Geometry check sheet. Reference: the model listing, model coordinates, mm. Round coordinates to 2 decimals unless told otherwise and drop trailing zeros. Loops run counter-clockwise (first coordinate to the right, second up) from the corner with the lowest first, then second, coordinate; pieces in that order, holes last. Notation, with made-up numbers: (62, 84.5) -> (74, 84.5) arc R16 ccw to (74, 107.5) -> close; hole circle Ø7 at (43.5, -29.5). An arc over 180 degrees is marked (long way). Use a Markdown table: item, result. Add a question column.
Q1. Sectioned sample at B-B, the plane y = 44.5. Enter the section's corners in (x, z).
Q2. Sectioned sample at A-A, the plane x = 13.75. Enter the section's corners in (y, z).
Q3. Material ranges on L1, parallel to Z at x = 18.5, y = 37; L2, parallel to Z at x = 12.5, y = 48; L3, parallel to X at y = 27, z = 25.5, recorded low to high.
Q4. Sectioned sample at C-C, the plane z = 31. Enter the section's corners in (x, y).
Q5. Gauge pin test, flat ends, axial feed: P1, Ø5.5, axis at y = 37, z = 24, coming from the -X side; P2, Ø1.5, axis at x = 19.5, y = 60, coming from the -Z side. Record the tip position at first contact, or that the pin passes through.
```python
from build123d import *

# Parameters (mm, degrees)
F1_DEPTH = 76.2
F2_R     = 5.08


with BuildPart() as f1:
    # F0 (on Front) → F1 (new body)
    with BuildSketch(Plane.XZ):
        Polygon((11.069345, -64.862475), (30.119345, -65.090583), (30.119345, 61.909417), (11.069345, 61.909417), (11.069345, 36.509417), (20.594345, 36.509417), (20.594345, 17.459417), (11.069345, 17.459417), align=None)
    extrude(amount=-F1_DEPTH)

    # F2
    f2_edges = [f1.edges().sort_by_distance(p)[0] for p in [
        (20.594345, 76.2, 61.909417),
        (30.119345, 38.1, 61.909417),
        (20.594345, 0, 61.909417),
        (11.069345, 38.1, 61.909417),
    ]]
    fillet(f2_edges, radius=F2_R)


solid = f1.part
```
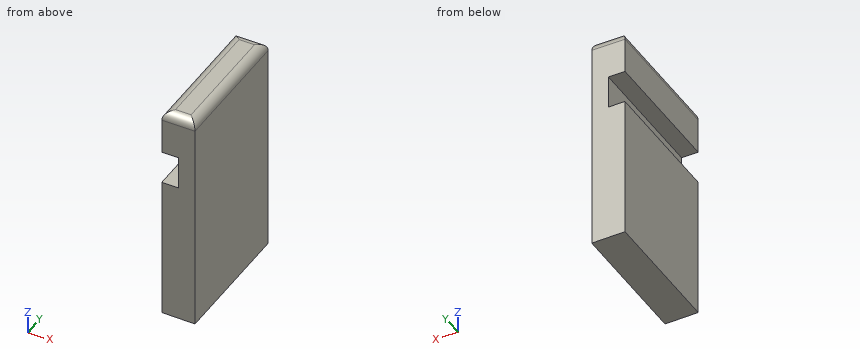
Values:
| question | item | result |
|---|---|---|
| 1 | outline | (11.07, -64.86) -> (30.12, -65.09) -> (30.12, 56.83) arc R5.08 ccw to (25.04, 61.91) -> (16.15, 61.91) arc R5.08 ccw to (11.07, 56.83) -> (11.07, 36.51) -> (20.59, 36.51) -> (20.59, 17.46) -> (11.07, 17.46) -> close |
| 2 | outline | (0, -64.89) -> (76.2, -64.89) -> (76.2, 17.46) -> (0, 17.46) -> close; (0, 36.51) -> (76.2, 36.51) -> (76.2, 56.83) arc R5.08 ccw to (73.52, 61.31) -> (2.68, 61.31) arc R5.08 ccw to (0, 56.83) -> close |
| 3 | L1 | -64.95 to 17.46, 36.51 to 61.91 |
| 3 | L2 | -64.88 to 17.46, 36.51 to 60.36 |
| 3 | L3 | 20.59 to 30.12 |
| 4 | outline | (20.59, 0) -> (30.12, 0) -> (30.12, 76.2) -> (20.59, 76.2) -> close |
| 5 | P1 | x = 20.59 |
| 5 | P2 | z = -64.97 |
